```python
from build123d import *

# Parameters (mm, degrees)
BOSS_EXTRU_1_DEPTH      = 20
CONG_1_R                = 0.5
CONG_2_R                = 1
BOSS_EXTRU_2_DEPTH      = 5
ENL_V_MAT_EXTRU_1_DEPTH = 35.78012648597392
ESQUISSE6_R             = 2.0500000000000007
ESQUISSE6_R_2           = 2.05
BOSS_EXTRU_3_DEPTH      = 5
CONG_4_R                = 1


with BuildPart() as part:
    # Esquisse1 → Boss.-Extru.1 (new body)
    with BuildSketch(Plane.XY):
        Polygon((-1.176e-14, 10.103135382441117), (-2.578e-14, 4.840000000000001), (3.5, 4.840000000000001), (5.71, 6.983135382441116), (5.71, 8.483135382441116), (2.95, 8.483135382441116), (2.95, 10.103135382441117), align=None)
        Polygon((-3.5, 4.840000000000001), (-2.576e-14, 4.840000000000001), (-1.176e-14, 10.103135382441117), (-2.95, 10.103135382441117), (-2.95, 8.483135382441116), (-5.71, 8.483135382441116), (-5.71, 6.983135382441116), align=None)
    extrude(amount=-BOSS_EXTRU_1_DEPTH)

    # Congé1
    cong_1_edges = [part.edges().sort_by_distance(p)[0] for p in [
        (5.71, 7.733135382441116, 0),
        (4.605, 5.911567691220558, 0),
        (0, 4.840000000000001, 0),
        (-4.605, 5.911567691220558, 0),
        (-5.71, 7.733135382441116, 0),
        (-5.71, 7.733135382441116, -20),
        (-4.605, 5.911567691220558, -20),
        (0, 4.840000000000001, -20),
        (4.605, 5.911567691220558, -20),
        (5.71, 7.733135382441116, -20),
    ]]
    fillet(cong_1_edges, radius=CONG_1_R)

    # Congé2
    # the kernel refuses this fillet: 1 mm, written as the material it takes off along each edge
    with BuildSketch(Plane(origin=(4.71, 7.4063748668930085, -20), x_dir=(1, 0, 0), z_dir=(0, 1, 0))) as cong_2_piece_1:
        with BuildLine():
            CenterArc((0.5, -0.5), 0.5, 0, 90)
            Line((1, -0.5), (1, 0))
            Line((1, 0), (0.5, 0))
        make_face()
    revolve(axis=Axis((4.71, 7.4063748668930085, -20), (0, 0, -1)), revolution_arc=45.87999999999987, mode=Mode.SUBTRACT)
    with BuildSketch(Plane(origin=(-4.710000000000001, 7.40637486689301, -20), x_dir=(-0.6961634275566162, -0.717883334625219, 0), z_dir=(0.717883334625219, -0.6961634275566162, 0))) as cong_2_piece_2:
        with BuildLine():
            CenterArc((0.5, -0.5), 0.5, 0, 90)
            Line((1, -0.5), (1, 0))
            Line((1, 0), (0.5, 0))
        make_face()
    revolve(axis=Axis((-4.710000000000001, 7.40637486689301, -20), (0, 0, -1)), revolution_arc=45.87999999999987, mode=Mode.SUBTRACT)
    with BuildSketch(Plane(origin=(4.71, 7.4063748668930085, 0), x_dir=(0.6961634275566162, -0.717883334625219, 0), z_dir=(-0.717883334625219, -0.6961634275566162, 0))) as cong_2_piece_3:
        with BuildLine():
            CenterArc((0.5, -0.5), 0.5, 0, 90)
            Line((1, -0.5), (1, 0))
            Line((1, 0), (0.5, 0))
        make_face()
    revolve(axis=Axis((4.71, 7.4063748668930085, 0), (0, 0, 1)), revolution_arc=45.87999999999987, mode=Mode.SUBTRACT)
    with BuildSketch(Plane(origin=(-4.710000000000001, 7.40637486689301, 0), x_dir=(-1, 0, 0), z_dir=(0, 1, 0))) as cong_2_piece_4:
        with BuildLine():
            CenterArc((0.5, -0.5), 0.5, 0, 90)
            Line((1, -0.5), (1, 0))
            Line((1, 0), (0.5, 0))
        make_face()
    revolve(axis=Axis((-4.710000000000001, 7.40637486689301, 0), (0, 0, 1)), revolution_arc=45.87999999999987, mode=Mode.SUBTRACT)
    with BuildSketch(Plane(origin=(-5.71, 6.983135382441116, 1.1e-16), x_dir=(0.717883334625219, -0.6961634275566161, 0), z_dir=(0, 0, -1))) as cong_2_piece_5:
        with BuildLine():
            CenterArc((CONG_2_R * 0.423239484452, -CONG_2_R), CONG_2_R, 90.00000000000003, 45.879999999999825)
            Line((-CONG_2_R * 0.294643850173, -CONG_2_R * 0.303836572443), (0, 0))
            Line((0, 0), (CONG_2_R * 0.423239484452, 0))
        make_face()
    extrude(amount=20, mode=Mode.SUBTRACT)
    with BuildSketch(Plane(origin=(5.71, 6.983135382441116, 1.1e-16), x_dir=(-0.7178833346252179, -0.6961634275566172, 0), z_dir=(0, 0, -1))) as cong_2_piece_6:
        with BuildLine():
            CenterArc((CONG_2_R * 0.423239484452, CONG_2_R), CONG_2_R, 224.12000000000015, 45.87999999999994)
            Line((-CONG_2_R * 0.294643850173, CONG_2_R * 0.303836572443), (0, 0))
            Line((0, 0), (CONG_2_R * 0.423239484452, 2e-17))
        make_face()
    extrude(amount=20, mode=Mode.SUBTRACT)

    # Esquisse3 → Boss.-Extru.2 (add)
    with BuildSketch(Plane(origin=(0, 10.103135382441117, 0), x_dir=(1, 0, 0), z_dir=(0, 1, 0))):
        Polygon((-10.550000000000004, 29.5), (10.549999999999994, 29.5), (10.55, -9.500000000000002), (-10.55, -9.500000000000002), align=None)
    extrude(amount=BOSS_EXTRU_2_DEPTH)

    # Esquisse5 → Enlèv. mat.-Extru.1 (cut, through all)
    with BuildSketch(Plane.XY):
        with BuildLine():
            Line((-5.209999999999999, 8.483135382441116), (-5.71, 8.483135382441116))
            Line((-5.71, 8.483135382441116), (-5.71, 7.4063748668930085))
            ThreePointArc((-5.71, 7.4063748668930085), (-5.630913521335368, 7.01660790289825), (-5.406163427556616, 6.68849153226779))
            Line((-5.406163427556616, 6.68849153226779), (-3.5, 4.840000000000001))
            Line((-3.5, 4.840000000000001), (3.5, 4.840000000000001))
            Line((3.5, 4.840000000000001), (5.406163427556617, 6.68849153226779))
            ThreePointArc((5.406163427556617, 6.68849153226779), (5.630913521335369, 7.01660790289825), (5.71, 7.406374866893009))
            Line((5.71, 7.406374866893009), (5.71, 8.483135382441116))
            Line((5.71, 8.483135382441116), (5.209999999999999, 8.483135382441116))
            Line((5.209999999999999, 8.483135382441116), (2.95, 8.483135382441116))
            Line((2.95, 8.483135382441116), (-2.95, 8.483135382441116))
            Line((-2.95, 8.483135382441116), (-5.209999999999999, 8.483135382441116))
        make_face()
    extrude(amount=-ENL_V_MAT_EXTRU_1_DEPTH, mode=Mode.SUBTRACT)

    # Esquisse6 → Boss.-Extru.3 (add)
    # profile 1 of 2: a face of its own
    with BuildSketch(Plane(origin=(0, 15.103135382441117, 0), x_dir=(1, 0, 0), z_dir=(0, 1, 0))):
        with BuildLine():
            ThreePointArc((-10.550000000000004, 29.5), (-4.56e-15, 40.05), (10.549999999999994, 29.5))
            Line((10.549999999999994, 29.5), (-10.550000000000004, 29.5))
        make_face()
        with Locations(Location((-5.53e-15, 34.775, 0), (0, 0, 270))):
            Circle(ESQUISSE6_R, mode=Mode.SUBTRACT)
    # profile 2 of 2: a face of its own
    with BuildSketch(Plane(origin=(0, 15.103135382441117, 0), x_dir=(1, 0, 0), z_dir=(0, 1, 0))):
        with BuildLine():
            ThreePointArc((-10.55, -9.500000000000002), (-1.94e-15, -20.050000000000004), (10.55, -9.500000000000002))
            Line((10.55, -9.500000000000002), (-10.55, -9.500000000000002))
        make_face()
        with Locations(Location((-9.7e-16, -14.775000000000002, 0), (0, 0, 270))):
            Circle(ESQUISSE6_R_2, mode=Mode.SUBTRACT)
    extrude(amount=-BOSS_EXTRU_3_DEPTH)

    # Congé4
    cong_4_edges = [part.edges().sort_by_distance(p)[0] for p in [
        (10.549999999999997, 10.103135382441117, -10),
        (-10.550000000000002, 10.103135382441117, -9.999999999999998),
        (10.549999999999997, 15.103135382441117, -10),
        (-10.550000000000002, 15.103135382441117, -9.999999999999998),
        (-8.32e-15, 15.103135382441117, -40.05),
        (-8.32e-15, 10.103135382441117, -40.05),
        (3.15e-15, 10.103135382441117, 20.050000000000004),
        (3.15e-15, 15.103135382441117, 20.050000000000004),
    ]]
    fillet(cong_4_edges, radius=CONG_4_R)


solid = part.part
```
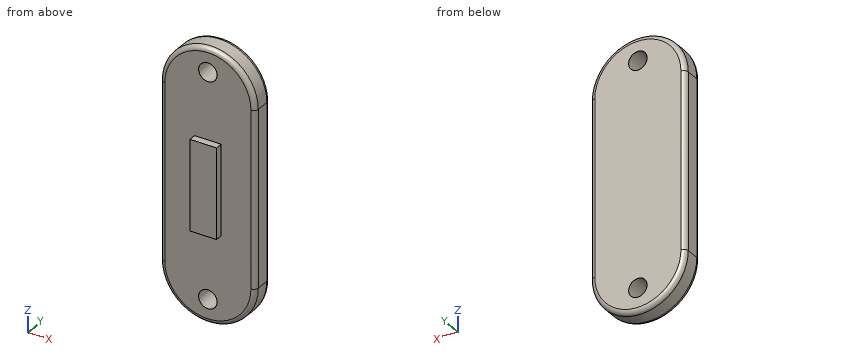
Model file for the job. Use its own axes, mm. Give positions to 0.01 mm unless a question says otherwise; leave off trailing zeros. Loops run counter-clockwise (first coordinate to the right, second up) from the corner with the lowest first, then second, coordinate; pieces in that order, holes last. Notation, with made-up numbers: M 0.25,66.25 L 13.25,66.25 A5 ccw 13.25,70.25 Z; hole C -12,0 d2. An arc over 180 degrees is marked long. Use one line per item in the form item = value.
Item 1: Slice it at D-D on z = -15.5. List the corners of the cut face in (x, y).
Filled in:
outline = M -10.55,11.1 A1 ccw -9.55,10.1 L -2.95,10.1 L -2.95,8.48 L 2.95,8.48 L 2.95,10.1 L 9.55,10.1 A1 ccw 10.55,11.1 L 10.55,14.1 A1 ccw 9.55,15.1 L -9.55,15.1 A1 ccw -10.55,14.1 Z
Item 2: Slice it at B-B on z = -26. List the corners of the cut face in (x, y), and give its area (3 significant figures).
Filled in:
outline = M -10.55,11.1 A1 ccw -9.55,10.1 L 9.55,10.1 A1 ccw 10.55,11.1 L 10.55,14.1 A1 ccw 9.55,15.1 L -9.55,15.1 A1 ccw -10.55,14.1 Z
area = 105 mm^2
Item 3: Slice it at A-A on x = 0. List the corners of the cut face in (y, z) (3 decimals), and give its area (3 significant figures).
Filled in:
outline = M 8.483,-20 L 10.103,-20 L 10.103,-32.725 L 15.103,-32.725 L 15.103,12.725 L 10.103,12.725 L 10.103,0 L 8.483,0 Z; M 10.103,-39.05 A1 ccw 11.103,-40.05 L 14.103,-40.05 A1 ccw 15.103,-39.05 L 15.103,-36.825 L 10.103,-36.825 Z; M 10.103,16.825 L 15.103,16.825 L 15.103,19.05 A1 ccw 14.103,20.05 L 11.103,20.05 A1 ccw 10.103,19.05 Z
area = 291 mm^2
Item 4: Drill centre lines: L1, parallel to Z at x = 0.25, y = 12.25; L2, parallel to Y at x = 1, z = -23; L3, parallel to X at y = 13.5, z = -35. Where is each one in solid material? Low to high.
Filled in:
L1 = -40.05 to -36.81, -32.74 to 12.74, 16.81 to 20.05
L2 = 10.1 to 15.1
L3 = -9 to -2.04, 2.04 to 9
Item 5: Slice it at C-C on y = 13. List the corners of the cut face in (x, z) (3 decimals), and give its area (3 significant figures).
Filled in:
outline = M -10.55,-29.5 A10.55 ccw 10.55,-29.5 L 10.55,9.5 A10.55 ccw -10.55,9.5 Z; hole C 0,-34.775 d4.1; hole C 0,14.775 d4.1
area = 1,150 mm^2
Item 6: Flat gauge pins, fed straight in: pin 1 Ø2 at (x, z) = (-7.5, -7) entering from -Y; pin 2 Ø3.5 at (x, z) = (0, 14.775) entering from -Y; pin 3 Ø1.8 at (y, z) = (9, -13.5) entering from -X; pin 4 Ø0.5 at (x, y) = (1, 9.5) entering from +Z. Where does each tip first touch, or does it go through?
Filled in:
pin_1 = 10.1
pin_2 = through
pin_3 = -2.95
pin_4 = 0
